from build123d import *

# Parameters (mm, degrees)
BOX001_W     = 4.7
BOX001_H     = 11
BOX001_DEPTH = 12
BOX002_W     = 4.7
BOX002_H     = 11
BOX002_DEPTH = 12
BOX_W        = 4.7
BOX_H        = 11
BOX_DEPTH    = 12
BOX003_W     = 45
BOX003_H     = 21
BOX003_DEPTH = 10


with BuildPart() as ranura2:
    # Box001 → Box001 (new body)
    with BuildSketch(Plane(origin=(15, 0, 0), x_dir=(1, 0, 0), z_dir=(0, 0, 1))):
        with Locations((2.35, 5.5)):
            Rectangle(BOX001_W, BOX001_H)
    extrude(amount=BOX001_DEPTH)


with BuildPart() as ranura3:
    # Box002 → Box002 (new body)
    with BuildSketch(Plane(origin=(30, 0, 0), x_dir=(1, 0, 0), z_dir=(0, 0, 1))):
        with Locations((2.35, 5.5)):
            Rectangle(BOX002_W, BOX002_H)
    extrude(amount=BOX002_DEPTH)


with BuildPart() as ranuras:
    # Box → Box (new body)
    with BuildSketch(Plane.XY):
        with Locations((2.35, 5.5)):
            Rectangle(BOX_W, BOX_H)
    extrude(amount=BOX_DEPTH)

    # Fusion: union ranura2, ranura3
    add(ranura2.part)
    add(ranura3.part)


with BuildPart() as ranuras_1:
    # Fusion placement: moved
    add(ranuras.part.moved(Location((5, 5, 2))))


with BuildPart() as cut:
    # Box003 → Box003 (new body)
    with BuildSketch(Plane.XY):
        with Locations((22.5, 10.5)):
            Rectangle(BOX003_W, BOX003_H)
    extrude(amount=BOX003_DEPTH)

    # Cut: cut ranuras
    add(ranuras_1.part, mode=Mode.SUBTRACT)


solid = cut.part
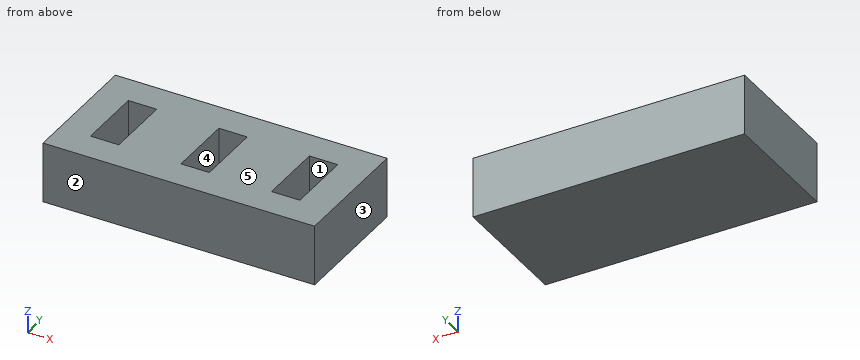
Can you work these out from the model? Positions are in its coordinate system, mm. Face numbers are marked on the shaded views. A direction names the side the tool comes from. Give positions to 0.01 mm unless a question says otherwise; leave off trailing zeros. Loops run counter-clockwise (first coordinate to the right, second up) from the corner with the lowest first, then second, coordinate; pieces in that order, holes last. Notation, with made-up numbers: (43.25, 80.5) - (68.25, 80.5) arc R20 cw to (68.25, 107.5) - close; hole circle Ø5 at (-13.75, 3.5). An arc over 180 degrees is marked (long way). One line per item, written item: value.
(1) If we mould it in two halves opening along X, with no side actions, what happens to the marked faces 1, 2 and 3? For each: released by +X, released by -X, zero draft, split by the parting line, or undercut.
Verdict:
face 1: undercut
face 2: zero draft
face 3: released by +X
(2) If we section it at C-C, the plane x = 7: List the corners of the cut face in (y, z) for me.
Verdict:
outline: (0, 0) - (21, 0) - (21, 10) - (16, 10) - (16, 2) - (5, 2) - (5, 10) - (0, 10) - close
(3) If we section it at A-A, the plane z = 2.5: List the corners of the cut face in (x, y) for me, plus the area to 3 significant figures.
Verdict:
outline: (0, 0) - (45, 0) - (45, 21) - (0, 21) - close; hole (5, 5) - (9.7, 5) - (9.7, 16) - (5, 16) - close; hole (20, 5) - (24.7, 5) - (24.7, 16) - (20, 16) - close; hole (35, 5) - (39.7, 5) - (39.7, 16) - (35, 16) - close
area: 790 mm^2
(4) On a 3-axis mill with a long thin cutter (end or side, diameter ignored), from which of +Z, -Z, +X, -X, +Y, -Y can I reach the whole of each face in a straight line? I mean the marked faces 4 and 5. Say none if no direction works.
Verdict:
face 4: +Z
face 5: +Z, +X, -X, +Y, -Y
(5) If we section it at B-B, the plane y = 13.25: List the corners of the cut face in (x, z) for me.
Verdict:
outline: (0, 0) - (45, 0) - (45, 10) - (39.7, 10) - (39.7, 2) - (35, 2) - (35, 10) - (24.7, 10) - (24.7, 2) - (20, 2) - (20, 10) - (9.7, 10) - (9.7, 2) - (5, 2) - (5, 10) - (0, 10) - close
(6) I need wall thicknesses on line 1 along X through (y, z) = (10, 5); line 2 along Y through (x, z) = (37.5, 9.75). Which ranges of each line are inside material? Lowest first, please.
Verdict:
line 1: 0 to 5, 9.7 to 20, 24.7 to 35, 39.7 to 45
line 2: 0 to 5, 16 to 21
(7) I'm going to push a flat-ended pin straight in: pin 1 (4 mm diameter, centred on x = 38, z = 8, fed in from -Y). Where does the tip first touch, or does it pass through?
Verdict:
pin 1: y = 0
